from build123d import *
from OCP.BRepFilletAPI import BRepFilletAPI_MakeChamfer

# Parameters (mm, degrees)
SKETCH2_R               = 4.765
BOSS_EXTRUDE1_DEPTH     = 9.5
CHAMFER1_SIZE           = 7.62
CHAMFER1_SIZE2          = 2.54
CHAMFER2_SIZE           = 2.54
CHAMFER2_SIZE2          = 7.62
SKETCH3_W               = 9.53
SKETCH3_H               = 9.53
CUT_EXTRUDE1_DEPTH      = 36.852041783
CUT_EXTRUDE2_DEPTH      = 32.648728647
CUT_EXTRUDE2_DEPTH_BACK = 32.648728647
CUT_EXTRUDE3_DEPTH      = 32.648728708
CUT_EXTRUDE3_DEPTH_BACK = 32.648728708
SKETCH5_R               = 1.59


with BuildPart() as part:
    # Sketch2 → Boss-Extrude1 (new, symmetric)
    with BuildSketch(Plane.XY):
        with BuildLine():
            Line((0, 9.725), (-22.23, 9.725))
            Line((-22.23, 9.725), (-22.23, 4.725))
            Line((-22.23, 4.725), (-9.658270439, -1.13729377))
            ThreePointArc((-9.658270439, -1.13729377), (-5.827126273, -7.785899075), (1.631914869, -9.587099606))
            Line((1.631914869, -9.587099606), (28.58, -5))
            Line((28.58, -5), (28.58, 0))
            Line((28.58, 0), (9.725, 0))
            ThreePointArc((9.725, 0), (6.876613447, 6.876613447), (0, 9.725))
        make_face()
        Circle(SKETCH2_R, mode=Mode.SUBTRACT)
    extrude(amount=BOSS_EXTRUDE1_DEPTH, both=True)

    # Chamfer1
    chamfer1_edges = [part.edges().sort_by_distance(p)[0] for p in [
        (-22.23, 7.225, -9.5),
        (28.58, -2.5, -9.5),
    ]]
    chamfer1_side = [part.faces().sort_by_distance(p)[0] for p in [
        (-11.115, 9.180944984, -9.5),
    ]]
    chamfer(chamfer1_edges, length=CHAMFER1_SIZE, length2=CHAMFER1_SIZE2, reference=chamfer1_side[0])

    # Chamfer2: one chamfer whose edges measure the first distance from different faces: ONE call of the kernel's chamfer builder (chamfer() names one face for all edges)
    chamfer2_edges_1 = [part.edges().sort_by_distance(p)[0] for p in [
        (-22.23, 7.225, 9.5),
    ]]
    chamfer2_side_1 = [part.faces().sort_by_distance(p)[0] for p in [
        (-22.23, 7.225, 1.27),
    ]]
    chamfer2_edges_2 = [part.edges().sort_by_distance(p)[0] for p in [
        (28.58, -2.5, 9.5),
    ]]
    chamfer2_side_2 = [part.faces().sort_by_distance(p)[0] for p in [
        (28.58, -2.5, 1.27),
    ]]
    chamfer2 = BRepFilletAPI_MakeChamfer(part.part.solid().wrapped)
    for e in chamfer2_edges_1:
        chamfer2.Add(CHAMFER2_SIZE, CHAMFER2_SIZE2, e.wrapped, chamfer2_side_1[0].wrapped)  # the first distance lies on this face
    for e in chamfer2_edges_2:
        chamfer2.Add(CHAMFER2_SIZE, CHAMFER2_SIZE2, e.wrapped, chamfer2_side_2[0].wrapped)  # the first distance lies on this face
    add(Compound.cast(chamfer2.Shape()), mode=Mode.REPLACE)

    # Sketch3 → Cut-Extrude1 (cut, through all)
    with BuildSketch(Plane(origin=(0, 9.725, 0), x_dir=(1, 0, 0), z_dir=(0, 1, 0))):
        with Locations((-17.465, 0)):
            Rectangle(SKETCH3_W, SKETCH3_H)
        with Locations((23.815, 0)):
            Rectangle(SKETCH3_W, SKETCH3_H)
    extrude(amount=-CUT_EXTRUDE1_DEPTH, mode=Mode.SUBTRACT)

    # Sketch4 → Cut-Extrude2 (cut, two sides: drawn at the far end of the back side and taken through both)
    with BuildSketch(Plane(origin=(0, 0, 0), x_dir=(1, 0, 0), z_dir=(0, 1, 0)).offset(-CUT_EXTRUDE2_DEPTH_BACK)):
        with BuildLine():
            Line((-3.72, 5.08), (6.44, 5.08))
            ThreePointArc((6.44, 5.08), (11.52, 0), (6.44, -5.08))
            Line((6.44, -5.08), (-3.72, -5.08))
            ThreePointArc((-3.72, -5.08), (-8.8, 0), (-3.72, 5.08))
        make_face()
    extrude(amount=CUT_EXTRUDE2_DEPTH + CUT_EXTRUDE2_DEPTH_BACK, mode=Mode.SUBTRACT)

    # Sketch5 → Cut-Extrude3 (cut, two sides: drawn at the far end of the back side and taken through both)
    with BuildSketch(Plane.XY.offset(-CUT_EXTRUDE3_DEPTH_BACK)):
        with Locations((-19.69, 7.275)):
            Circle(SKETCH5_R)
        with Locations((26.13, -2.45)):
            Circle(SKETCH5_R)
    extrude(amount=CUT_EXTRUDE3_DEPTH + CUT_EXTRUDE3_DEPTH_BACK, mode=Mode.SUBTRACT)


solid = part.part
CAD build for the part. Positions are in the model's coordinates, mm. A direction names the side the tool comes from. Round coordinates to 2 decimals unless told otherwise and drop trailing zeros. Write each loop counter-clockwise with the first axis right and the second up, starting at its lowest first coordinate (ties: lowest second). Pieces come first, ordered by that corner, then holes.
(1) 3-axis set-ups, long thin cutter, end or side, ignore diameter. For faces 1 (the face through (23.977, -3.193, -8.494)), 2 (the face through (5, 0, 5.08)), 3 (the face through (-17.52, 6.46, 8.53)), 4 (the face through (-16, 6, 4.765)), 5 (the face through (23, -3, 4.765)): which of +Z, -Z, +X, -X, +Y, -Y reach the whole face in a straight line?
(2) Slice it at B-B, the plane z = -0.25. Write the cut outline in (x, y) (3 decimals), and give its area (3 significant figures).
(3) Slice it at D-D, the plane x = -19.69. Write the cut outline in (y, z) (3 decimals), and give its area (3 significant figures).
(4) Probe line 1 along Z through (x, y) = (6.5, -7.75); line 2 along Z through (x, y) = (-14, 1.75) (3 decimals); line 3 along X through (y, z) = (-1, 7.75). List the from-to ranges inside material, lowest first.
(5) Mould opens along Y. For faces 6 (the face through (28.58, -3, 6)), 7 (the face through (-0.62, 4.724, -7.267)), 8 (the face through (-11, 9.725, 0)) say: pulls with the +Y half, pulls with the -Y half, needs draft (parallel to the pull), parting line crosses it, or undercut.
(6) Slice it at A-A, the plane y = 3.5. Write the cut outline in (x, z) (3 decimals), and give its area (3 significant figures).
(7) Slice it at C-C, the plane x = -13.5. Write the cut outline in (y, z) (3 decimals), and give its area (3 significant figures).
(8) Drop flat-ended pins along their axis: P1, Ø3.5, axis at x = -19.69, y = 7.275, coming from the -Z side; P2, Ø1, axis at y = -5, z = 2, coming from the -X side; P3, Ø9.5, axis at x = 22.5, z = -4, coming from the +Y side. Give the stop position or say it passes through.
From the geometry:
1. face 1: -Z, +X, +Y, -Y
1. face 2: +Y, -Y
1. face 3: +Z, -X, +Y, -Y
1. face 4: -X, +Y, -Y
1. face 5: +X, +Y, -Y
2. outline: (-12.7, 0.281) - (-9.658, -1.137) arc R9.725 ccw to (-8.794, -4.153) - (-8.794, 9.725) - (-12.7, 9.725) - close; (11.514, -7.905) - (19.05, -6.622) - (19.05, 0) - (11.514, 0) - close
2. area: 96.6 mm2
3. outline: (3.541, -7.807) - (5.685, -7.807) - (5.685, -4.765) - (3.541, -4.765) - close; (3.541, 4.765) - (5.685, 4.765) - (5.685, 7.807) - (3.541, 7.807) - close; (8.865, -7.807) - (9.725, -7.807) - (9.725, -4.765) - (8.865, -4.765) - close; (8.865, 4.765) - (9.725, 4.765) - (9.725, 7.807) - (8.865, 7.807) - close
3. area: 18.3 mm2
4. line 1: z = -9.5 to -5.08, 5.08 to 9.5
4. line 2: z = -9.5 to -4.765, 4.765 to 9.5
4. line 3: x = -9.95 to -4.66, 4.66 to 25.48
5. face 6: needs draft
5. face 7: undercut
5. face 8: pulls with the +Y half
6. outline: (-19.603, -7.836) - (-14.61, -9.5) - (-3.233, -9.5) - (-3.233, -5.08) - (-3.72, -5.08) arc R5.08 cw to (-3.72, 5.08) - (-3.233, 5.08) - (-3.233, 9.5) - (-14.61, 9.5) - (-19.603, 7.836) - (-19.603, 4.765) - (-12.7, 4.765) - (-12.7, -4.765) - (-19.603, -4.765) - close; (3.233, -9.5) - (9.073, -9.5) - (9.073, -4.344) arc R5.08 cw to (6.44, -5.08) - (3.233, -5.08) - close; (3.233, 5.08) - (6.44, 5.08) arc R5.08 cw to (9.073, 4.344) - (9.073, 9.5) - (3.233, 9.5) - close
6. area: 244 mm2
7. outline: (0.654, -9.5) - (9.725, -9.5) - (9.725, -4.765) - (0.654, -4.765) - close; (0.654, 4.765) - (9.725, 4.765) - (9.725, 9.5) - (0.654, 9.5) - close
7. area: 85.9 mm2
8. P1: stops at z = -8.39
8. P2: stops at x = -8.62
8. P3: stops at y = 0
